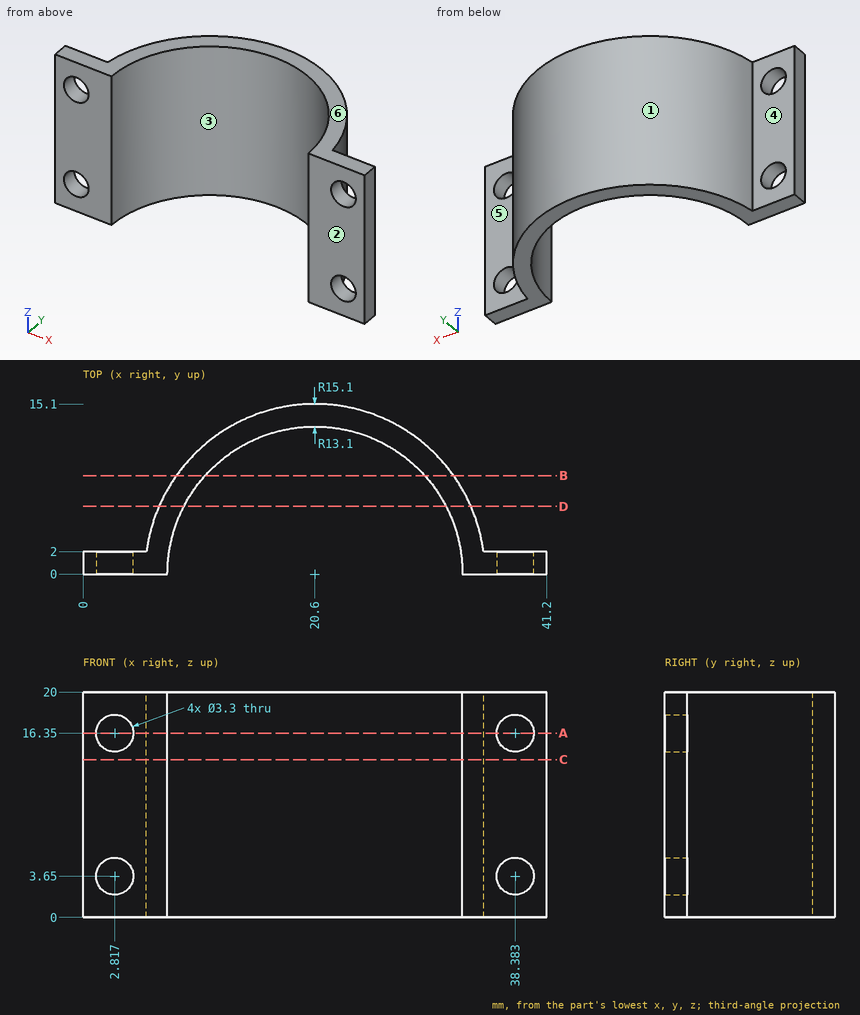
The figure shows three views and two pictorial views of one solid part (mm, origin at its lowest corner). Answer the questions. A direction names the side the tool comes from. Coordinates: 2 decimals unless noted, no trailing zeros. Order: outer loops, then holes, each group sorted by start corner. A loop starts at its lowest first (then second) coordinate and runs counter-clockwise, first axis right, second up.
Q1. Consider line 1 (X direction, y = 3, z = 8.25); line 2 (X direction, y = 8, z = 14.5) (1 decimal); line 3 (Z direction, x = 38, y = 1.75) (1 decimal). Determine where each line is inside the solid, lowest interval first.
Q2. Which of the six approach directions +Z, -Z, +X, -X, +Y, -Y give full straight-line access (tool end or side, diameter ignored) to the marked faces 4, 5 and 6?
Q3. A cutting plane is placed at D-D, the plane y = 6. Write down the section's boundary in (x, z) (1 decimal).
Q4. A cutting plane is placed at C-C, the plane z = 14. Write down the section's boundary in (x, y).
Q5. Given P1, Ø5.5, axis at x = 38.38, z = 16.35, coming from the +Y side; P2, Ø1, axis at y = 4.5, z = 3, coming from the -X side, each flat-ended and moving along its own axis, determine where each tip first touches the part or whether it passes through.
Q6. For a pull along X with two mould halves and no side action, classify the marked faces 1, 2 and 3 as pulls with the +X half, pulls with the -X half, needs draft (parallel to the pull), parting line crosses it, or undercut.
Q7. A cutting plane is placed at B-B, the plane y = 8.75. Write down the section's boundary in (x, z), and give its area (3 significant figures).
Q8. A cutting plane is placed at A-A, the plane z = 16.35. Write down the section's boundary in (x, y).
Answers follow:
1. line 1: x = 5.8 to 7.85, 33.35 to 35.4
1. line 2: x = 7.8 to 10.2, 31 to 33.4
1. line 3: z = 0 to 2, 5.3 to 14.7, 18 to 20
2. face 4: +Z, -Z, -X, +Y
2. face 5: +Z, -Z, +X, +Y
2. face 6: +Z, +X, -X, +Y, -Y
3. outline: (6.7, 0) - (9, 0) - (9, 20) - (6.7, 20) - close; (32.2, 0) - (34.5, 0) - (34.5, 20) - (32.2, 20) - close
4. outline: (0, 0) - (7.5, 0) arc R13.1 cw to (33.7, 0) - (41.2, 0) - (41.2, 2) - (35.57, 2) arc R15.1 ccw to (5.63, 2) - (0, 2) - close
5. P1: stops at y = 2
5. P2: stops at x = 6.04
6. face 1: parting line crosses it
6. face 2: needs draft
6. face 3: undercut
7. outline: (8.29, 0) - (10.85, 0) - (10.85, 20) - (8.29, 20) - close; (30.35, 0) - (32.91, 0) - (32.91, 20) - (30.35, 20) - close
7. area: 102 mm2
8. outline: (0, 0) - (1.17, 0) - (1.17, 2) - (0, 2) - close; (4.47, 0) - (7.5, 0) arc R13.1 cw to (33.7, 0) - (36.73, 0) - (36.73, 2) - (35.57, 2) arc R15.1 ccw to (5.63, 2) - (4.47, 2) - close; (40.03, 0) - (41.2, 0) - (41.2, 2) - (40.03, 2) - close
